Geometry: final body of the model. Coordinates: model frame, mm. A direction names the side the tool comes from. Give positions to 0.01 mm unless a question says otherwise; leave off trailing zeros. Write each loop counter-clockwise with the first axis right and the second up, starting at its lowest first coordinate (ties: lowest second). Pieces come first, ordered by that corner, then holes.
Autodesk Inventor part; units mm, degrees
ref_plane "YZ Plane" through (0, 0, 0) normal (1, 0, 0) x (0, 1, 0)
ref_plane "XZ Plane" through (0, 0, 0) normal (0, 1, 0) x (-1, 0, 0)
ref_plane "XY Plane" through (0, 0, 0) normal (0, 0, 1) x (1, 0, 0)
sketch "Sketch1" plane through (0, 0, 0) normal (0, 1, 0) x (-1, 0, 0)
  circle A0 centre (0, 0) radius 25
  dimension "d0" = 50
extrude "Extrusion1" add sketch "Sketch1" along normal blind 5
sketch "Sketch2" plane through (0, 5, 0) normal (0, 1, 0) x (1, 0, 0)
  circle A0 centre (0, 0) radius 25
extrude "Extrusion2" add sketch "Sketch2" along normal blind 25
sketch "Sketch3" plane through (0, 30, 0) normal (0, 1, 0) x (1, 0, 0)
  circle A0 centre (0, 0) radius 25
  line L0 (0, 25) -> (21.6506, 12.5)
  line L1 (21.6506, 12.5) -> (21.6506, -12.5)
  line L2 (21.6506, -12.5) -> (0, -25)
  line L3 (0, -25) -> (-21.6506, -12.5)
  line L4 (-21.6506, -12.5) -> (-21.6506, 12.5)
  line L5 (-21.6506, 12.5) -> (0, 25)
  point P0 (0, -25)
extrude "Extrusion3" cut sketch "Sketch3" against normal blind 25 contours A0 L1 | L5 A0 | A0 L3
sketch "Sketch4" plane through (0, 30, 0) normal (0, 1, 0) x (1, 0, 0)
  arc A0 (-21.6506, 12.5) -> (-21.6506, -12.5) centre (0, 0) ccw
  line L0 (-21.6506, 12.5) -> (0, 25)
  line L1 (0, 25) -> (21.6506, 12.5)
  line L2 (21.6506, 12.5) -> (21.6506, -12.5)
  line L3 (21.6506, -12.5) -> (0, -25)
  line L4 (0, -25) -> (-21.6506, -12.5)
  line L5 (-21.6506, -12.5) -> (-21.6506, 12.5)
  circle A1 centre (0, 0) radius 25
  line L6 (-18.6506, 10.7679) -> (0, 21.5359)
  line L7 (0, 21.5359) -> (18.6506, 10.7679)
  line L8 (18.6506, 10.7679) -> (18.6506, -10.7679)
  line L9 (18.6506, -10.7679) -> (0, -21.5359)
  line L10 (0, -21.5359) -> (-18.6506, -10.7679)
  line L11 (-18.6506, -10.7679) -> (-18.6506, 10.7679)
  dimension "d7" = 3
extrude "Extrusion4" cut sketch "Sketch4" against normal blind 25 contours L6 L7 L8 L9 L10 L11
sketch "Sketch5" plane through (0, 5, -25) normal (-0.5, 0, -0.8660254) x (-0.8660254, 0, 0.5)
  circle A0 centre (12.5, 12.5) radius 5.5
  line L0 (0, 0) -> (0, 25)
  line L1 (0, 0) -> (25, 0)
  line L2 (0, 25) -> (25, 25)
  line L3 (25, 25) -> (25, 0)
  point P0 (12.5, -5)
  point P1 (25, 12.5)
  dimension "d10" = 11
  dimension "d11" = 12.5
  dimension "d12" = 12.5
  dimension "d13" = 12.5
  dimension "d14" = 12.5
extrude "Extrusion5" cut sketch "Sketch5" against normal blind 25 contours A0
pattern_circular "Circular Pattern1" count 3 over 360 about axis through (0, 0, 0) along (0, 1, 0) of "Extrusion5"
sketch "Sketch6" plane through (0, 0, 0) normal (0, -1, 0) x (1, 0, 0)
  circle A0 centre (0, 0) radius 12
  circle A1 centre (0, 0) radius 13.2
  dimension "d20" = 24
  dimension "d21" = 26.4
extrude "Extrusion6" add sketch "Sketch6" along normal blind 10
sketch "Sketch7" plane through (0, 0, 0) normal (0, -1, 0) x (1, 0, 0)
  circle A0 centre (0, 0) radius 12
extrude "Extrusion7" cut sketch "Sketch7" against normal blind 10
properties part number "spojkaV2"
Q1. Section D-D on x = 3. Output: boundary loops of the cut face in (y, z), plus the area to 3 significant figures.
Filled sheet:
outline: (-10, -12.85) - (0, -12.85) - (0, -24.82) - (30, -24.82) - (30, -19.8) - (5, -19.8) - (5, -11.62) - (-10, -11.62) - close; (-10, 11.62) - (5, 11.62) - (5, 19.8) - (30, 19.8) - (30, 24.82) - (0, 24.82) - (0, 12.85) - (-10, 12.85) - close
area: 407 mm2
Q2. Access query for faces 4 (the flat face through (-11, 0, -11)), 5 (the flat face through (18.651, 20.5, -4.9)), 6 (the cylindrical face through (20.17, 21.22, 4.05)), 7 (the flat face through (23, 5, 0)). Directions: +Z, -Z, +X, -X, +Y, -Y. A direction counts if a zero-diameter tool reaches every point of the face in a straight line with its end or side. Return the directions, or none.
Filled sheet:
face 4: -Y
face 5: +Y
face 6: +X
face 7: +Z, -Z, +X, +Y
Q3. Pin query (flat end, axial travel): P1, Ø6, axis at x = -15.5, z = -2.5, coming from the +Y side; P2, Ø10, axis at y = 5, z = -5.5, coming from the +X side (3 decimals); P3, Ø17, axis at y = 19.5, z = -2, coming from the +X side. Return the tip coordinate at first contact, or that it passes through.
Filled sheet:
P1: stops at y = 5
P2: stops at x = 24.995
P3: stops at x = 21.65
Q4. Section C-C on z = -2. Output: boundary loops of the cut face in (x, y), plus the area to 3 significant figures.
Filled sheet:
outline: (-24.92, 0) - (-13.05, 0) - (-13.05, -10) - (-11.83, -10) - (-11.83, 5) - (-18.65, 5) - (-18.65, 30) - (-24.92, 30) - close; (11.83, -10) - (13.05, -10) - (13.05, 0) - (24.92, 0) - (24.92, 5) - (21.65, 5) - (21.65, 12.38) - (18.65, 12.38) - (18.65, 5) - (11.83, 5) - close; (18.65, 22.62) - (21.65, 22.62) - (21.65, 30) - (18.65, 30) - close
area: 356 mm2
Q5. Section B-B on y = 17.5. Output: boundary loops of the cut face in (x, z).
Filled sheet:
outline: (-21.65, -12.5) - (-15.59, -16) - (-14.09, -13.4) - (-18.65, -10.77) - (-18.65, 10.77) - (-14.09, 13.4) - (-15.59, 16) - (-21.65, 12.5) arc R25 ccw to start; (-6.06, -21.5) - (0, -25) arc R25 ccw to (21.65, -12.5) - (21.65, -5.5) - (18.65, -5.5) - (18.65, -10.77) - (0, -21.54) - (-4.56, -18.9) - close; (-6.06, 21.5) - (-4.56, 18.9) - (0, 21.54) - (18.65, 10.77) - (18.65, 5.5) - (21.65, 5.5) - (21.65, 12.5) arc R25 ccw to (0, 25) - close
Q6. Section A-A on y = 25. Output: boundary loops of the cut face in (x, z), plus the area to 3 significant figures.
Filled sheet:
outline: (-21.65, -12.5) - (0, -25) arc R25 ccw to (21.65, -12.5) - (21.65, 12.5) arc R25 ccw to (0, 25) - (-21.65, 12.5) arc R25 ccw to start; hole (-18.65, -10.77) - (0, -21.54) - (18.65, -10.77) - (18.65, 10.77) - (0, 21.54) - (-18.65, 10.77) - close
area: 589 mm2
Q7. Pull-direction query (Z, two-part tool) for faces 1 (the cylindrical face through (-11.99, -2.61, 0.53)), 2 (the flat face through (21.651, 23.2, -0.2)), 3 (the flat face through (-5.863, 17.675, 21.615)); classes: released by +Z, released by -Z, zero draft, split by the parting line, or undercut.
Filled sheet:
face 1: undercut
face 2: zero draft
face 3: released by +Z
Q8. Ray query, line 1 along Y through (x, z) = (20, 0); line 2 along Z through (x, y) = (0, -1.25); line 3 along Y through (x, z) = (8, 11). Return the intervals inside material, ascending.
Filled sheet:
line 1: y = 0 to 12, 23 to 30
line 2: z = -13.2 to -12, 12 to 13.2
line 3: y = 0 to 5
